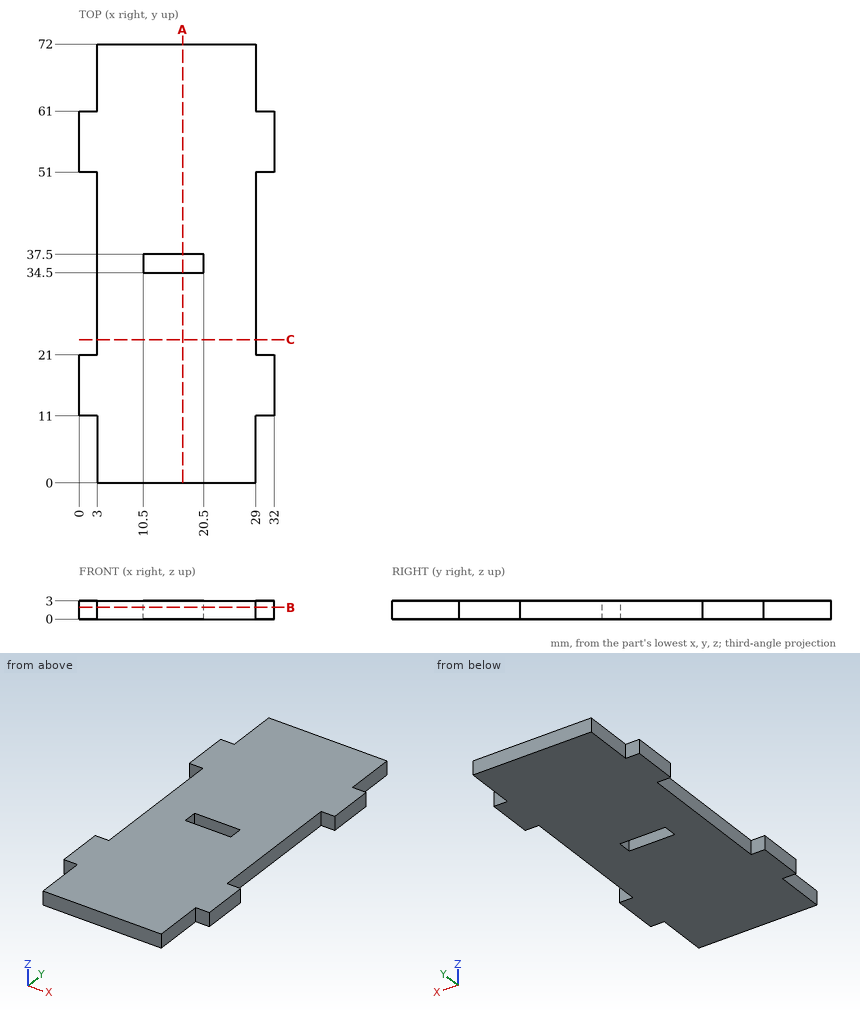
The figure shows three views and two pictorial views of one solid part (mm, origin at its lowest corner). Answer the questions. Coordinates: 2 decimals unless noted, no trailing zeros. Order: outer loops, then holes, each group sorted by start corner. A loop starts at its lowest first (then second) coordinate and runs counter-clockwise, first axis right, second up. Notation, with made-up numbers: (-37, 3) - (-12, 3) arc R38 cw to (-12, 42) - close; hole circle Ø10 at (40.5, 75). An arc over 180 degrees is marked (long way). Answer as a JSON object with one key per item and string values.
1. Find section C-C on y = 23.5. Determine the outline of the cut face in (x, z), plus the area to 3 significant figures.
Output values:
{"outline": "(3, 0) - (29, 0) - (29, 3) - (3, 3) - close", "area": "78.0 mm²"}
2. Find section A-A on x = 17. Determine the outline of the cut face in (y, z), plus the area to 3 significant figures.
Output values:
{"outline": "(0, 0) - (34.5, 0) - (34.5, 3) - (0, 3) - close; (37.5, 0) - (72, 0) - (72, 3) - (37.5, 3) - close", "area": "207 mm²"}
3. Consider line 1 (Y direction, x = 19, z = 2.3); line 2 (Y direction, x = 30, z = 2.6); line 3 (X direction, y = 9, z = 1.2). Determine where each line is inside the solid, lowest interval first.
Output values:
{"line 1": "y = 0 to 34.5, 37.5 to 72", "line 2": "y = 11 to 21, 51 to 61", "line 3": "x = 3 to 29"}
4. Each of these flat-tipped pins is pushed along its axis until it touches: P1, Ø1.5, axis at x = 1, z = 2, coming from the -Y side; P2, Ø0.9, axis at y = 64, z = 1, coming from the +X side; P3, Ø1.5, axis at x = 2, z = 1.5, coming from the +Y side. Where does it stop, or does it pass through?
Output values:
{"P1": "stops at y = 11", "P2": "stops at x = 29", "P3": "stops at y = 61"}
5. Find section B-B on z = 1.95. Determine the outline of the cut face in (x, y).
Output values:
{"outline": "(0, 11) - (3, 11) - (3, 0) - (29, 0) - (29, 11) - (32, 11) - (32, 21) - (29, 21) - (29, 51) - (32, 51) - (32, 61) - (29, 61) - (29, 72) - (3, 72) - (3, 61) - (0, 61) - (0, 51) - (3, 51) - (3, 21) - (0, 21) - close; hole (10.5, 34.5) - (20.5, 34.5) - (20.5, 37.5) - (10.5, 37.5) - close"}
